Geometry: final body of the model. Coordinates: model frame, mm. Round coordinates to 2 decimals unless told otherwise and drop trailing zeros. Order: outer loops, then holes, each group sorted by start corner. A loop starts at its lowest first (then second) coordinate and runs counter-clockwise, first axis right, second up. Notation, with made-up numbers: (-10.5, 5) -> (12.5, 5) arc R20 ccw to (12.5, 22) -> close; hole circle Ø9 at (-38.5, 4). An arc over 180 degrees is marked (long way). Put each result on its own line as item: value.
Autodesk Inventor part; units mm, degrees
ref_plane "YZ Plane" through (0, 0, 0) normal (1, 0, 0) x (0, 1, 0)
ref_plane "XZ Plane" through (0, 0, 0) normal (0, 1, 0) x (-1, 0, 0)
ref_plane "XY Plane" through (0, 0, 0) normal (0, 0, 1) x (1, 0, 0)
sketch "Boceto1" plane through (0, 0, 0) normal (0, 1, 0) x (-1, 0, 0)
  circle A0 centre (-88.569, 59.1067) radius 3.5
  circle A1 centre (-29.569, 59.1067) radius 3.5
  line L0 (-88.569, 59.1067) -> (-29.569, 59.1067)
  circle A2 centre (-29.569, -25.8933) radius 3.5
  line L1 (-29.569, 59.1067) -> (-29.569, -25.8933)
  circle A3 centre (-88.569, -25.8933) radius 3.5
  line L2 (-29.569, -25.8933) -> (-88.569, -25.8933)
  line L3 (-88.569, -25.8933) -> (-88.569, 59.1067)
  line L4 (-96.569, 66.6067) -> (-21.569, 66.6067)
  line L5 (-21.569, 66.6067) -> (-21.569, 51.6067)
  line L6 (-96.569, 51.6067) -> (-96.569, 66.6067)
  line L7 (-96.569, 66.6067) -> (-21.569, 51.6067) construction
  line L8 (-21.569, 66.6067) -> (-96.569, 51.6067) construction
  line L9 (-37.569, -33.3933) -> (-21.569, -33.3933)
  line L10 (-21.569, -33.3933) -> (-21.569, 66.6067)
  line L11 (-21.569, 66.6067) -> (-37.569, 66.6067)
  line L12 (-37.569, -33.3933) -> (-21.569, 66.6067) construction
  line L13 (-21.569, -33.3933) -> (-37.569, 66.6067) construction
  line L14 (-21.569, -18.3933) -> (-21.569, -33.3933)
  line L15 (-21.569, -33.3933) -> (-96.569, -33.3933)
  line L16 (-96.569, -33.3933) -> (-96.569, -18.3933)
  line L17 (-96.569, -18.3933) -> (-21.569, -33.3933) construction
  line L18 (-21.569, -18.3933) -> (-96.569, -33.3933) construction
  line L19 (-80.569, -33.3933) -> (-96.569, -33.3933)
  line L20 (-96.569, -33.3933) -> (-96.569, 66.6067)
  line L21 (-96.569, 66.6067) -> (-80.569, 66.6067)
  line L22 (-80.569, -33.3933) -> (-96.569, 66.6067) construction
  line L23 (-96.569, -33.3933) -> (-80.569, 66.6067) construction
  line L24 (-80.569, -18.3933) -> (-37.569, -18.3933)
  line L25 (-80.569, 51.6067) -> (-80.569, -18.3933)
  line L26 (-37.569, 51.6067) -> (-37.569, -18.3933)
  circle A4 centre (-88.569, 59.1067) radius 3.5
  circle A5 centre (-29.569, 59.1067) radius 3.5
  circle A6 centre (-29.569, -25.8933) radius 3.5
  circle A7 centre (-88.569, -25.8933) radius 3.5
  line L27 (-37.569, 51.6067) -> (-80.569, 51.6067)
  point P0 (0, 0)
  point P1 (-59.069, 59.1067)
  point P2 (-29.569, 16.6067)
  point P3 (-59.069, -25.8933)
  point P4 (-88.569, 16.6067)
  dimension "d0" = 75
  dimension "d1" = 15
extrude "Extrusión1" add sketch "Boceto1" along normal blind 5 contours L0 A1 L1 A2 L2 A3 L3 A0 | L4 L5 L10 L9 L15 L16 L20 L6
properties part number "jetson_union"
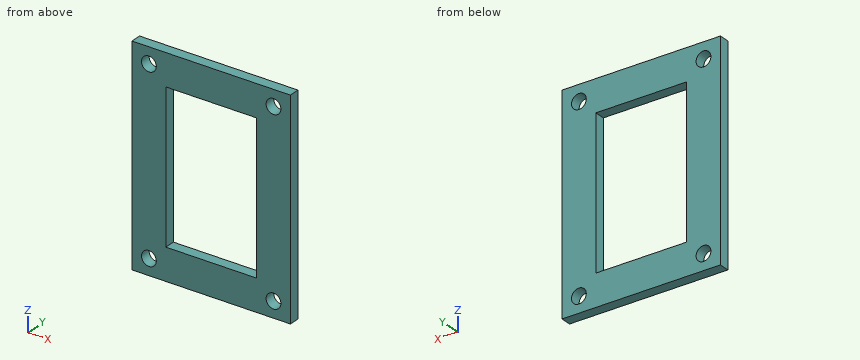
1. Cut plane B-B on z = -5. Return loops of the section in (x, y), and give its area (3 significant figures).
Ans:
outline: (21.57, 0) -> (37.57, 0) -> (37.57, 5) -> (21.57, 5) -> close; (80.57, 0) -> (96.57, 0) -> (96.57, 5) -> (80.57, 5) -> close
area: 160 mm²
2. Material intervals for probe 1 along X at (y, z) = (3.4, 11); probe 2 along Z at (x, y) = (52, 0.8); probe 3 along Z at (x, y) = (29, 4.4), sorted ascending.
Ans:
probe 1: 21.57 to 37.57, 80.57 to 96.57
probe 2: -33.39 to -18.39, 51.61 to 66.61
probe 3: -33.39 to -29.35, -22.44 to 55.65, 62.56 to 66.61
3. Cut plane A-A on x = 48.5. Return loops of the section in (y, z).
Ans:
outline: (0, -33.39) -> (5, -33.39) -> (5, -18.39) -> (0, -18.39) -> close; (0, 51.61) -> (5, 51.61) -> (5, 66.61) -> (0, 66.61) -> close
4. Cut plane C-C on y = 2.8. Return loops of the section in (x, z), and give its area (3 significant figures).
Ans:
outline: (21.57, -33.39) -> (96.57, -33.39) -> (96.57, 66.61) -> (21.57, 66.61) -> close; hole circle Ø7 at (29.57, -25.89); hole circle Ø7 at (29.57, 59.11); hole (37.57, -18.39) -> (80.57, -18.39) -> (80.57, 51.61) -> (37.57, 51.61) -> close; hole circle Ø7 at (88.57, -25.89); hole circle Ø7 at (88.57, 59.11)
area: 4,340 mm²
5. Contact query for flat-ended pins moving along their axis: P1, Ø5, axis at x = 84.5, z = -22, coming from the -Y side; P2, Ø4, axis at x = 88.57, z = 59.11, coming from the -Y side. Output: stop coordinate, or through.
Ans:
P1: y = 0
P2: through
